Source: CAD feature listing. Evaluate the final solid. Frame: model axes, mm. A direction names the side the tool comes from. Give positions to 0.01 mm unless a question says otherwise; leave off trailing zeros. Write each loop counter-clockwise with the first axis right and the second up, starting at its lowest first coordinate (ties: lowest second). Pieces come first, ordered by that corner, then holes.
```python
from build123d import *

# Parameters (mm, degrees)
SKETCH1_R             = 4.95
SKETCH1_W             = 5
SKETCH1_H             = 10
SKETCH1_W_2           = 8.5
BODY_DEPTH            = 3
SKETCH1_3_R           = 4.95
SKETCH1_3_R_2         = 2.5
MOUNT_INSETS_DEPTH    = 1.5
SKETCH1_5_W           = 5
SKETCH1_5_H           = 10
HINGE_DEPTH           = 15
SKETCH2_R             = 4.95
SKETCH2_R_2           = 2.5
HINGE_INSET_DEPTH     = 1.5
HINGE_START           = -17
SKETCH2_2_R           = 4.95
SKETCH2_2_R_2         = 2.5
HINGE_INSET2_DEPTH    = 1.5
SKETCH2_3_R           = 2.5
HINGE_SCREWHOLE_DEPTH = 120.897733068


with BuildPart() as part:
    # Sketch1 → Body (new body)
    # profile 1 of 4: a face of its own
    with BuildSketch(Plane.XY):
        Polygon((-23.27588231, 115.303529412), (-34.02588231, 115.303529412), (-34.02588231, 90.303529412), (-24.02588231, 90.303529412), (-24.02588231, -29.696470588), (-34.02588231, -29.696470588), (-34.02588231, -54.696470588), (5.97411769, -54.696470588), (5.97411769, -29.696470588), (-4.02588231, -29.696470588), (-4.02588231, 90.303529412), (5.97411769, 90.303529412), (5.97411769, 115.303529412), (-4.77588231, 115.303529412), (-4.77588231, 105.303529412), (-9.77588231, 105.303529412), (-18.27588231, 105.303529412), (-23.27588231, 105.303529412), align=None)
        with Locations((-14.02588231, -49.696470588)):
            Circle(SKETCH1_R, mode=Mode.SUBTRACT)
        with Locations((-14.02588231, -39.696470588)):
            Circle(SKETCH1_R, mode=Mode.SUBTRACT)
    # profile 2 of 4: a face of its own
    with BuildSketch(Plane.XY):
        with Locations((-20.77588231, 110.303529412)):
            Rectangle(SKETCH1_W, SKETCH1_H)
    # profile 3 of 4: a face of its own
    with BuildSketch(Plane.XY):
        with Locations((-14.02588231, 110.303529412)):
            Rectangle(SKETCH1_W_2, SKETCH1_H)
    # profile 4 of 4: a face of its own
    with BuildSketch(Plane.XY):
        with Locations((-7.27588231, 110.303529412)):
            Rectangle(SKETCH1_W, SKETCH1_H)
    extrude(amount=BODY_DEPTH)

    # Sketch1<3> → Mount Insets (add)
    # profile 1 of 2: a face of its own
    with BuildSketch(Plane.XY):
        with Locations((-14.02588231, -39.696470588)):
            Circle(SKETCH1_3_R)
        with Locations((-14.02588231, -39.696470588)):
            Circle(SKETCH1_3_R_2, mode=Mode.SUBTRACT)
    # profile 2 of 2: a face of its own
    with BuildSketch(Plane.XY):
        with Locations((-14.02588231, -49.696470588)):
            Circle(SKETCH1_3_R)
        with Locations((-14.02588231, -49.696470588)):
            Circle(SKETCH1_3_R_2, mode=Mode.SUBTRACT)
    extrude(amount=MOUNT_INSETS_DEPTH)

    # Sketch1<5> → Hinge (add)
    with BuildSketch(Plane.XY):
        with Locations((-7.27588231, 110.303529412)):
            Rectangle(SKETCH1_5_W, SKETCH1_5_H)
        with Locations((-20.77588231, 110.303529412)):
            Rectangle(SKETCH1_5_W, SKETCH1_5_H)
    extrude(amount=HINGE_DEPTH)

    # Sketch2 → Hinge Inset (cut)
    with BuildSketch(Plane(origin=(-4.77588231, 0, 0), x_dir=(0, 0, -1), z_dir=(1, 0, 0))):
        with Locations((-10, 110.303529412)):
            Circle(SKETCH2_R)
        with Locations((-10, 110.303529412)):
            Circle(SKETCH2_R_2, mode=Mode.SUBTRACT)
    extrude(amount=-HINGE_INSET_DEPTH, mode=Mode.SUBTRACT)

    # Sketch2<2> → Hinge Inset2 (cut)
    with BuildSketch(Plane(origin=(-4.77588231, 0, 0), x_dir=(0, 0, -1), z_dir=(1, 0, 0)).offset(HINGE_START)):
        with Locations((-10, 110.303529412)):
            Circle(SKETCH2_2_R)
        with Locations((-10, 110.303529412)):
            Circle(SKETCH2_2_R_2, mode=Mode.SUBTRACT)
    extrude(amount=-HINGE_INSET2_DEPTH, mode=Mode.SUBTRACT)

    # Sketch2<3> → Hinge Screwhole (cut, through all)
    with BuildSketch(Plane(origin=(-4.77588231, 0, 0), x_dir=(0, 0, -1), z_dir=(1, 0, 0))):
        with Locations(Location((-10, 110.303529412, 0), (0, 0, 270))):
            Circle(SKETCH2_3_R)
    extrude(amount=-HINGE_SCREWHOLE_DEPTH, mode=Mode.SUBTRACT)


solid = part.part
```
1. Cut plane A-A, the plane z = 10. Return the cut outline in (x, y), then the cut area to 3 significant figures.
2. Mould query, pull axis X, two halves, no side actions, for faces 6 (the flat face through (-24.026, 31, 1)), 7 (the cylindrical face through (-15, -52, 1)), 8 (the flat face through (-18.276, 109.1, 7.6)), 9 (the flat face through (-21, 110, 15)). Classes: +X half, -X half, draft (parallel to the pull), parting line (faces both ways), or undercut.
3. Contact query for flat-ended pins moving along their axis: P1, Ø0.9, axis at y = 21, z = 2, coming from the -X side; P2, Ø2, axis at x = -16.5, y = -35, coming from the -Z side; P3, Ø8, axis at x = -14.03, y = -49.7, coming from the +Z side; P4, Ø11, axis at x = -13.5, y = -39, coming from the +Z side. Output: stop coordinate, or through.
4. Access query for faces 1 (the flat face through (-4.776, 110.2, 4.9)), 2 (the flat face through (-29, -29.696, 1)), 3 (the flat face through (-23.276, 110.2, 4.9)), 4 (the flat face through (-6.276, 113, 11)), 5 (the cylindrical face through (-22.52, 105.91, 7.72)). Directions: +Z, -Z, +X, -X, +Y, -Y. A direction counts if a zero-diameter tool reaches every point of the face in a straight line with its end or side. Return the directions, or none.
5. Line query: L1, parallel to Y at x = -25.5, z = 1.5; L2, parallel to Y at x = -20.55, z = 10; L3, parallel to Z at x = -26.5, y = 95. Output: solid intervals per line, ascending.
6. Cut plane B-B, the plane x = -1.5. Return the cut outline in (y, z).
7. Cut plane C-C, the plane y = 25.5. Return the cut outline in (x, z).
Response values:
1. outline: (-23.28, 105.3) - (-18.28, 105.3) - (-18.28, 107.8) - (-21.78, 107.8) - (-21.78, 105.35) - (-23.28, 105.35) - close; (-23.28, 115.25) - (-21.78, 115.25) - (-21.78, 112.8) - (-18.28, 112.8) - (-18.28, 115.3) - (-23.28, 115.3) - close; (-9.78, 105.3) - (-4.78, 105.3) - (-4.78, 105.35) - (-6.28, 105.35) - (-6.28, 107.8) - (-9.78, 107.8) - close; (-9.78, 112.8) - (-6.28, 112.8) - (-6.28, 115.25) - (-4.78, 115.25) - (-4.78, 115.3) - (-9.78, 115.3) - close
1. area: 35.3 mm2
2. face 6: -X half
2. face 7: undercut
2. face 8: undercut
2. face 9: draft
3. P1: stops at x = -24.03
3. P2: stops at z = 0
3. P3: stops at z = 1.5
3. P4: stops at z = 3
4. face 1: +Z, +X, +Y, -Y
4. face 2: +Z, -Z, -X
4. face 3: +Z, -X, +Y, -Y
4. face 4: +X
4. face 5: -X
5. L1: y = -54.7 to -29.7, 90.3 to 115.3
5. L2: y = 105.3 to 107.8, 112.8 to 115.3
5. L3: z = 0 to 3
6. outline: (-54.7, 0) - (-29.7, 0) - (-29.7, 3) - (-54.7, 3) - close; (90.3, 0) - (115.3, 0) - (115.3, 3) - (90.3, 3) - close
7. outline: (-24.03, 0) - (-4.03, 0) - (-4.03, 3) - (-24.03, 3) - close
